from build123d import *

# Parameters (mm, degrees)
F0_W     = 30
F0_H     = 26
F0_R     = 1.45
F1_DEPTH = 22
F2_R     = 6.25
F3_DEPTH = 26.001
F4_R     = 1.5
F5_DEPTH = 13


# Not quite as in the source:
# - a feature names something its author has since deleted; it is built from what else it names


with BuildPart() as f1:
    # F0 (on Top) → F1 (new body)
    with BuildSketch(Plane.XY):
        Rectangle(F0_W, F0_H)
        with Locations((-12, -10)):
            Circle(F0_R, mode=Mode.SUBTRACT)
        with Locations((12, -10)):
            Circle(F0_R, mode=Mode.SUBTRACT)
        with Locations((-12, 10)):
            Circle(F0_R, mode=Mode.SUBTRACT)
        with Locations((12, 10)):
            Circle(F0_R, mode=Mode.SUBTRACT)
    extrude(amount=F1_DEPTH)

    # F2 (on face) → F3 (cut, through all)
    with BuildSketch(Plane(origin=(0, 13, 0), x_dir=(-1, 0, 0), z_dir=(0, 1, 0))):
        with Locations((0, 11)):
            Circle(F2_R)
    extrude(amount=-F3_DEPTH, mode=Mode.SUBTRACT)

    # F4 (on face) → F5 (cut)
    with BuildSketch(Plane(origin=(-15, 0, 0), x_dir=(0, -1, 0), z_dir=(-1, 0, 0))):
        with Locations((0, 11)):
            Circle(F4_R)
    extrude(amount=-F5_DEPTH, mode=Mode.SUBTRACT)


solid = f1.part
Model file for the job. Use its own axes, mm. A direction names the side the tool comes from. Coordinates: 2 decimals unless noted, no trailing zeros. Write each loop counter-clockwise with the first axis right and the second up, starting at its lowest first coordinate (ties: lowest second). Pieces come first, ordered by that corner, then holes. Notation, with made-up numbers: (63.5, 45.25) -> (94.5, 45.25) arc R17 cw to (94.5, 53.25) -> close; hole circle Ø5 at (69.25, 70.25). An arc over 180 degrees is marked (long way). One line per item, written item: value. Start each with the question number.
1) Pull direction X, two halves, no side cores. Call faces 1 (the face through (-15, 0, 8)), 2 (the face through (10.85, 9.12, 10.85)), 3 (the face through (0, 0, 0)), 4 (the face through (15, 0, 11)): +X half, -X half, draft (parallel to the pull), parting line (faces both ways), or undercut.
2) Slice it at D-D on z = 10.25. Write the cut outline in (x, y).
3) Which spindle directions (+Z, -Z, +X, -X, +Y, -Y) get a long thin tool onto all of the face, cutting with end or side? Do faces 5 (the face through (-10.596, 0.325, 9.536)), 6 (the face through (0, 0, 22)). Say none if no direction does.
4) Flat gauge pins, fed straight in: pin 1 Ø2.5 at (y, z) = (0, 11) entering from -X; pin 2 Ø4.5 at (x, y) = (12, -10) entering from -Z; pin 3 Ø2.5 at (x, y) = (-12, -10) entering from -Z. Where does each tip first touch, or does it go through?
5) Slice it at B-B on x = -12. Write the cut outline in (y, z), then the cut area to 3 significant figures.
6) Slice it at A-A on y = -10. Write the cut outline in (x, z), then the cut area to 3 significant figures.
7) Probe probe 1 along Y at (x, z) = (-12, 8.25); probe 2 along Z at (x, y) = (0, -10.75); probe 3 along X at (y, z) = (-2.25, 15). List the from-to ranges inside material, lowest first.
8) Slice it at C-C on z = 16.5. Write the cut outline in (x, y), then the cut area to 3 significant figures.
Answers follow:
1. face 1: -X half
1. face 2: undercut
1. face 3: draft
1. face 4: +X half
2. outline: (-15, -13) -> (-6.2, -13) -> (-6.2, -1.3) -> (-15, -1.3) -> close; (-15, 1.3) -> (-6.2, 1.3) -> (-6.2, 13) -> (-15, 13) -> close; (6.2, -13) -> (15, -13) -> (15, 13) -> (6.2, 13) -> close; hole circle Ø2.9 at (-12, -10); hole circle Ø2.9 at (-12, 10); hole circle Ø2.9 at (12, -10); hole circle Ø2.9 at (12, 10)
3. face 5: -X
3. face 6: +Z, +X, -X, +Y, -Y
4. pin 1: x = 6.12
4. pin 2: z = 0
4. pin 3: through
5. outline: (-13, 0) -> (-11.45, 0) -> (-11.45, 22) -> (-13, 22) -> close; (-8.55, 0) -> (8.55, 0) -> (8.55, 22) -> (-8.55, 22) -> close; (11.45, 0) -> (13, 0) -> (13, 22) -> (11.45, 22) -> close; hole circle Ø3 at (0, 11)
5. area: 437 mm2
6. outline: (-15, 0) -> (-13.45, 0) -> (-13.45, 22) -> (-15, 22) -> close; (-10.55, 0) -> (10.55, 0) -> (10.55, 22) -> (-10.55, 22) -> close; (13.45, 0) -> (15, 0) -> (15, 22) -> (13.45, 22) -> close; hole circle Ø12.5 at (0, 11)
6. area: 410 mm2
7. probe 1: -13 to -11.45, -8.55 to 8.55, 11.45 to 13
7. probe 2: 0 to 4.75, 17.25 to 22
7. probe 3: -15 to -4.8, 4.8 to 15
8. outline: (-15, -13) -> (-2.97, -13) -> (-2.97, 13) -> (-15, 13) -> close; (2.97, -13) -> (15, -13) -> (15, 13) -> (2.97, 13) -> close; hole circle Ø2.9 at (-12, -10); hole circle Ø2.9 at (-12, 10); hole circle Ø2.9 at (12, -10); hole circle Ø2.9 at (12, 10)
8. area: 599 mm2
